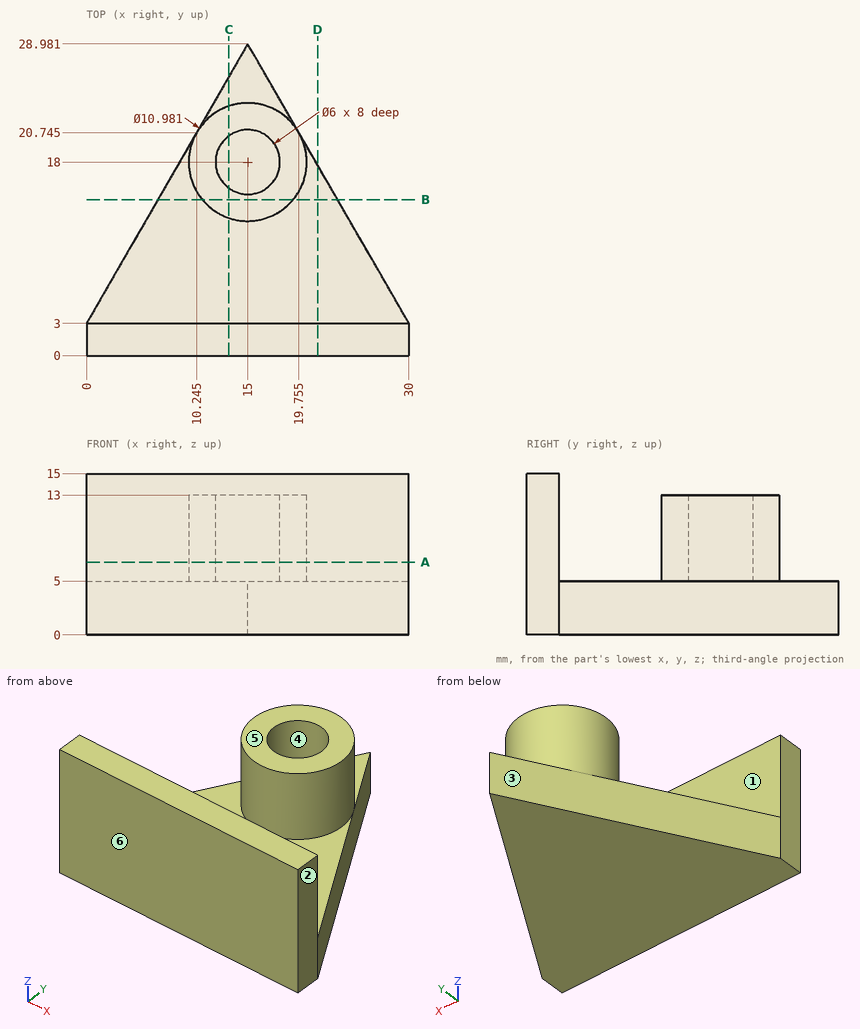
Design review of the part shown in the three views and the two pictorial views. Dimensions are in mm from the part's minimum x, y and z. A direction names the side the tool comes from. Round coordinates to 2 decimals unless told otherwise and drop trailing zeros. Order: outer loops, then holes, each group sorted by start corner. A loop starts at its lowest first (then second) coordinate and runs counter-clockwise, first axis right, second up.
(1) Take a section at B-B, the plane y = 14.5. State the section outline as (x, z) points, plus the area to 3 significant figures.
Working result:
outline: (6.64, 0) - (23.36, 0) - (23.36, 5) - (19.23, 5) - (19.23, 13) - (10.77, 13) - (10.77, 5) - (6.64, 5) - close
area: 151 mm2
(2) Wall thickness on L1, parallel to Y at x = 15, z = 8.25; L2, parallel to Y at x = 24, z = 11; L3, parallel to Z at x = 26.5, y = 7.5: over which ranges is each line inside the solid? List them lowest first.
Working result:
L1: y = 0 to 3, 12.51 to 15, 21 to 23.49
L2: y = 0 to 3
L3: z = 0 to 5
(3) Take a section at D-D, the plane x = 21.5. State the section outline as (y, z) points.
Working result:
outline: (0, 0) - (17.72, 0) - (17.72, 5) - (3, 5) - (3, 15) - (0, 15) - close
(4) Take a section at A-A, the plane z = 6.75. State the section outline as (x, y) points, plus the area to 3 significant figures.
Working result:
outline: (0, 0) - (30, 0) - (30, 3) - (0, 3) - close; circle Ø10.98 at (15, 18); hole circle Ø6 at (15, 18)
area: 156 mm2
(5) Mouldability with a two-part tool opening along Y and no side actions: class the marked faces 1, 2 and 3 as released by +Y, released by -Y, zero draft, split by the parting line, or undercut.
Working result:
face 1: undercut
face 2: zero draft
face 3: released by +Y
(6) Take a section at C-C, the plane x = 13.25. State the section outline as (y, z) points, plus the area to 3 significant figures.
Working result:
outline: (0, 0) - (25.95, 0) - (25.95, 5) - (23.2, 5) - (23.2, 13) - (20.44, 13) - (20.44, 5) - (15.56, 5) - (15.56, 13) - (12.8, 13) - (12.8, 5) - (3, 5) - (3, 15) - (0, 15) - close
area: 204 mm2
(7) For P1, Ø1, axis at x = 9.5, z = 8.5, coming from the -Y side; P2, Ø9, axis at x = 10.5, y = 11, coming from the +Z side; P3, Ø6, axis at x = 24.5, y = 6.5, coming from the +Z side; P4, Ø1, axis at y = 9.5, z = 2, coming from the -X side, all flat-tipped, find the tip position at first contact; note any pin that passes through.
Working result:
P1: stops at y = 0
P2: stops at z = 13
P3: stops at z = 5
P4: stops at x = 3.46
(8) Tool access review of the marked faces 4, 5 and 6: name each direction out of +Z, -Z, +X, -X, +Y, -Y from which nothing blocks a thin tool from reaching the whole face with its end or side.
Working result:
face 4: +Z
face 5: +Z, +X, -X, +Y
face 6: +Z, -Z, +X, -X, -Y
